from build123d import *

# Parameters (mm, degrees)
F1_DEPTH = 6


with BuildPart() as f1:
    # F0 (on Top) → F1 (new body)
    with BuildSketch(Plane.XY):
        with BuildLine():
            Line((18, 0), (9.5, 0))
            ThreePointArc((9.5, 0), (6.7175144213, -6.7175144213), (0, -9.5))
            Line((0, -9.5), (0, -18))
            Line((0, -18), (18, -18))
            Line((18, -18), (40, -18))
            Line((40, -18), (60.1537041366, -18))
            ThreePointArc((60.1537041366, -18), (78.1537041366, 0), (60.1537041366, 18))
            Line((60.1537041366, 18), (40, 18))
            Line((40, 18), (18, 18))
            Line((18, 18), (18, 0))
        make_face()
        Polygon((35.8430780618, -7.2), (31.6861561237, 0), (35.8430780618, 7.2), (44.1569219382, 7.2), (48.3138438763, 0), (44.1569219382, -7.2), align=None, mode=Mode.SUBTRACT)
        with BuildLine():
            ThreePointArc((0, 9.5), (6.7175144213, 6.7175144213), (9.5, 0))
            Line((9.5, 0), (18, 0))
            Line((18, 0), (18, 18))
            Line((18, 18), (0, 18))
            Line((0, 18), (0, 9.5))
        make_face()
        with BuildLine():
            ThreePointArc((-9.5, 0), (-6.7175144213, 6.7175144213), (0, 9.5))
            Line((0, 9.5), (0, 18))
            Line((0, 18), (-18, 18))
            Line((-18, 18), (-18, 0))
            Line((-18, 0), (-9.5, 0))
        make_face()
        with BuildLine():
            Line((0, -18), (0, -9.5))
            ThreePointArc((0, -9.5), (-6.7175144213, -6.7175144213), (-9.5, 0))
            Line((-9.5, 0), (-18, 0))
            Line((-18, 0), (-18, -18))
            Line((-18, -18), (0, -18))
        make_face()
        Polygon((0, 40), (0, 18), (18, 18), (18, 58), (6.2353829072, 58), (6.2353829072, 54.4), (0, 50.8), align=None)
        Polygon((-18, 18), (0, 18), (0, 40), (0, 50.8), (-6.2353829072, 54.4), (-6.2353829072, 58), (-18, 58), (-18, 40), align=None)
        Polygon((0, -50.8), (0, -18), (-18, -18), (-18, -58), (-6.2353829072, -58), (-6.2353829072, -54.4), align=None)
        Polygon((18, -18), (0, -18), (0, -50.8), (6.2353829072, -54.4), (6.2353829072, -58), (18, -58), align=None)
        with BuildLine():
            Line((-18, -18), (-18, 0))
            Line((-18, 0), (-18, 18))
            Line((-18, 18), (-40, 18))
            Line((-40, 18), (-60, 18))
            ThreePointArc((-60, 18), (-78, 0), (-60, -18))
            Line((-60, -18), (-40, -18))
            Line((-40, -18), (-18, -18))
        make_face()
        Polygon((-36.4, 6.2353829072), (-32.8, 0), (-36.4, -6.2353829072), (-43.6, -6.2353829072), (-47.2, 0), (-43.6, 6.2353829072), align=None, mode=Mode.SUBTRACT)
        with BuildLine():
            Line((6.2353829072, 58), (18, 58))
            ThreePointArc((18, 58), (0, 76), (-18, 58))
            Line((-18, 58), (-6.2353829072, 58))
            Line((-6.2353829072, 58), (-6.2353829072, 61.6))
            Line((-6.2353829072, 61.6), (0, 65.2))
            Line((0, 65.2), (6.2353829072, 61.6))
            Line((6.2353829072, 61.6), (6.2353829072, 58))
        make_face()
        with BuildLine():
            Line((-6.2353829072, -58), (-18, -58))
            ThreePointArc((-18, -58), (0, -76), (18, -58))
            Line((18, -58), (6.2353829072, -58))
            Line((6.2353829072, -58), (6.2353829072, -61.6))
            Line((6.2353829072, -61.6), (0, -65.2))
            Line((0, -65.2), (-6.2353829072, -61.6))
            Line((-6.2353829072, -61.6), (-6.2353829072, -58))
        make_face()
    extrude(amount=F1_DEPTH)


solid = f1.part
The model under review builds one solid part; all positions refer to its coordinate system, in mm. A direction names the side the tool comes from. Coordinates: 2 decimals unless noted, no trailing zeros. Loops run counter-clockwise (first coordinate to the right, second up) from the corner with the lowest first, then second, coordinate; pieces in that order, holes last. Notation, with made-up numbers: M -24.75,80 L 33.25,80 A19 ccw 33.25,96 Z; hole C 54.5,13.5 d3. An arc over 180 degrees is marked long. Put each result on its own line as item: value. Start each with the question number.
Q1. The part is to be moulded in two halves that separate along X. For faces 1 (the flat face through (18, 38, 3)), 2 (the cylindrical face through (0, -76, 3)), 3 (the flat face through (-40, -6.235, 3)), say which applies: +X half, -X half, draft (parallel to the pull), parting line (faces both ways), or undercut.
Q2. Clearance check with flat-ended pins moving along their axes: pin 1 (3 mm diameter, centred on x = -49, z = 3.5, fed in from +Y); pin 2 (1.5 mm diameter, centred on y = 35.5, z = 1, fed in from -X); pin 3 (1.8 mm diameter, centred on x = -39, z = 2.5, fed in from -Y). State where each tip first meets the part, or that it passes through.
Q3. For faces 4 (the flat face through (-18, -38, 3)), 5 (the flat face through (-45.375, -3.161, 2.958)), 6 (the flat face through (-18, 38, 3)), 7 (the flat face through (18, -38, 3)), list the 3-axis set-ups (+Z, -Z, +X, -X, +Y, -Y) from which the entire face can be reached by the end or side of a thin tool; tool diameter is ignored.
Q4. Add section B-B (z = 1.9). Count the separate pieces of the cut face and the enclosed holes in it, and give its area (3 significant figures).
Q5. Add section A-A (y = 45). Write out the cut boundary in (x, z), and give its area (3 significant figures).
Q6. Wall thickness on line 1 (X direction, y = -56.5, z = 1.1); line 2 (Y direction, x = 43, z = 2.2); line 3 (X direction, y = -6, z = 1.3): over which ranges is each line inside the solid? List them lowest first.
Answers:
1. face 1: +X half
1. face 2: parting line
1. face 3: undercut
2. pin 1: stops at y = 18
2. pin 2: stops at x = -18
2. pin 3: stops at y = -18
3. face 4: +Z, -Z, -X, -Y
3. face 5: +Z, -Z
3. face 6: +Z, -Z, -X, +Y
3. face 7: +Z, -Z, +X, -Y
4. separate pieces: 1
4. enclosed holes: 5
4. area: 8,370 mm^2
5. outline: M -18,0 L 18,0 L 18,6 L -18,6 Z
5. area: 216 mm^2
6. line 1: x = -18 to -6.24, 6.24 to 18
6. line 2: y = -18 to -7.2, 7.2 to 18
6. line 3: x = -76.97 to -43.74, -36.26 to -7.37, 7.37 to 35.15, 44.85 to 77.12
